The drawing under review shows one solid part. Ordinate dimensions are in mm from its lowest x, y, z. A direction names the side the tool comes from. Give positions to 0.01 mm unless a question says otherwise; leave off trailing zeros. Loops run counter-clockwise (first coordinate to the right, second up) from the corner with the lowest first, then second, coordinate; pieces in that order, holes last. Notation, with made-up numbers: M -28.75,-32.75 L -1.75,-32.75 A21 cw -1.75,-7.75 Z; hole C 89.5,17.5 d11. An arc over 180 degrees is marked long. Answer as CSV lines item,"result".
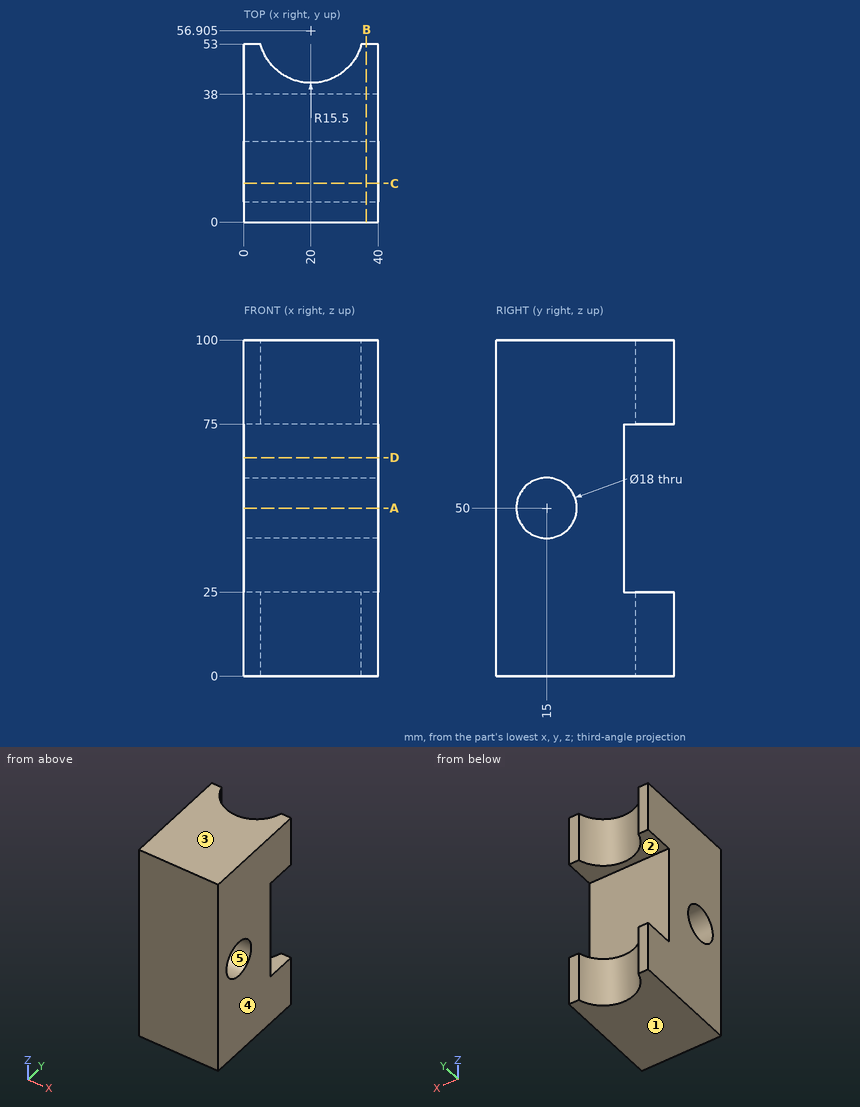
1. We need section B-B, the plane x = 36.5. Write out the cut boundary in (y, z), plus the area to 3 significant figures.
Answer block:
outline,"M 0,0 L 53,0 L 53,25 L 38,25 L 38,75 L 53,75 L 53,100 L 0,100 Z; hole C 15,50 d18"
area,"4,300 mm²"
2. To check wall thickness, follow L1, parallel to Y at x = 21, z = 50; L2, parallel to Y at x = 6, z = 72.5; L3, parallel to Z at x = 35, y = 48. State the ranges of each line that lie inside material, in increasing order. Write a range as [from, to].
Answer block:
L1,"[0, 6], [24, 38]"
L2,"[0, 38]"
L3,"[0, 25], [75, 100]"
3. For P1, Ø2, axis at x = 8.5, z = 75.5, coming from the +Y side; P2, Ø12, axis at x = 27.5, z = 40, coming from the +Y side; P3, Ø6, axis at y = 41.5, z = 65, coming from the -X side, all flat-tipped, find the tip position at first contact; note any pin that passes through.
Answer block:
P1,"y = 47.74"
P2,"y = 38"
P3,"through"
4. We need section D-D, the plane z = 65. Write out the cut boundary in (x, y).
Answer block:
outline,"M 0,0 L 40,0 L 40,38 L 0,38 Z"
5. We need section C-C, the plane y = 11.5. Write out the cut boundary in (x, z).
Answer block:
outline,"M 0,0 L 40,0 L 40,41.71 L 0,41.71 Z; M 0,58.29 L 40,58.29 L 40,100 L 0,100 Z"
6. We need section A-A, the plane z = 50. Write out the cut boundary in (x, y).
Answer block:
outline,"M 0,0 L 40,0 L 40,6 L 0,6 Z; M 0,24 L 40,24 L 40,38 L 0,38 Z"
7. For the marked faces 1 and 2, list the 3-axis set-ups (+Z, -Z, +X, -X, +Y, -Y) from which the entire face can be reached by the end or side of a thin tool; tool diameter is ignored.
Answer block:
face 1,"-Z, +X, -X, +Y, -Y"
face 2,"+X, -X, +Y"
8. The part is to be moulded in two halves that separate along Z. For the marked faces 3, 4 and 5, say which applies: pulls with the +Z half, pulls with the -Z half, needs draft (parallel to the pull), parting line crosses it, or undercut.
Answer block:
face 3,"pulls with the +Z half"
face 4,"needs draft"
face 5,"undercut"
